Can you work these out from the model? Positions are in its coordinate system, mm. Face numbers are marked on the shaded views. A direction names the side the tool comes from. Give positions to 0.01 mm unless a question says otherwise; leave off trailing zeros. Order: outer loops, then holes, each group sorted by start corner. A loop starts at its lowest first (then second) coordinate and runs counter-clockwise, first axis right, second up. Notation, with made-up numbers: (56, 85.5) - (104, 85.5) arc R28 cw to (104, 110.5) - close; hole circle Ø1 at (31.5, 71.5). An arc over 180 degrees is marked (long way). Write each question's results on one line, items separated by ' | '. Start each with the question number.
from build123d import *

# Parameters (mm, degrees)
BOSS_EXTRUDE1_DEPTH = 25.4
SKETCH2_R           = 6.35
SKETCH2_R_2         = 6.289382054
CUT_EXTRUDE1_DEPTH  = 6.35
SKETCH3_R           = 6.35
CUT_EXTRUDE2_DEPTH  = 65.834626806


with BuildPart() as part:
    # Sketch1 → Boss-Extrude1 (new body)
    with BuildSketch(Plane.XY):
        with BuildLine():
            Line((1.27, 42.381959669), (0, 42.400983542))
            Line((0, 42.400983542), (-1.27, 42.381959669))
            ThreePointArc((-1.27, 42.381959669), (-4.039167101, 38.714670348), (-4.477654975, 34.140282326))
            ThreePointArc((-4.477654975, 34.140282326), (-5.686801313, 32.251452896), (-7.469044916, 33.61281957))
            ThreePointArc((-7.469044916, 33.61281957), (-9.445621582, 37.761366553), (-13.302074292, 40.260380337))
            Line((-13.302074292, 40.260380337), (-14.501990468, 39.843891349))
            Line((-14.501990468, 39.843891349), (-15.688893549, 39.391649173))
            ThreePointArc((-15.688893549, 39.391649173), (-17.036772621, 34.998413532), (-15.884283593, 30.549923177))
            ThreePointArc((-15.884283593, 30.549923177), (-16.374491771, 28.361451696), (-18.514867758, 29.031154701))
            ThreePointArc((-18.514867758, 29.031154701), (-21.7911289, 32.253484654), (-26.269722106, 33.282804957))
            Line((-26.269722106, 33.282804957), (-27.25482686, 32.481037825))
            Line((-27.25482686, 32.481037825), (-28.215474992, 31.650124428))
            ThreePointArc((-28.215474992, 31.650124428), (-27.979491926, 27.060831521), (-25.375033182, 23.274792424))
            ThreePointArc((-25.375033182, 23.274792424), (-25.08717686, 21.050640851), (-27.327524299, 20.947904121))
            ThreePointArc((-27.327524299, 20.947904121), (-31.50830447, 22.855356494), (-36.068853735, 22.290832097))
            Line((-36.068853735, 22.290832097), (-36.720328893, 21.200491771))
            Line((-36.720328893, 21.200491771), (-37.338853735, 20.091127572))
            ThreePointArc((-37.338853735, 20.091127572), (-35.547471572, 15.859313854), (-31.805179274, 13.192378205))
            ThreePointArc((-31.805179274, 13.192378205), (-30.773978173, 11.200812045), (-32.844078098, 10.338027146))
            ThreePointArc((-32.844078098, 10.338027146), (-37.425113508, 10.700535032), (-41.517549284, 8.610255909))
            Line((-41.517549284, 8.610255909), (-41.756817328, 7.362853523))
            Line((-41.756817328, 7.362853523), (-41.958615655, 6.108844216))
            ThreePointArc((-41.958615655, 6.108844216), (-38.827901521, 2.744928878), (-34.399151351, 1.518768476))
            ThreePointArc((-34.399151351, 1.518768476), (-32.748983542, 0), (-34.399151351, -1.518768476))
            ThreePointArc((-34.399151351, -1.518768476), (-38.827901521, -2.744928878), (-41.958615655, -6.108844216))
            Line((-41.958615655, -6.108844216), (-41.756817328, -7.362853523))
            Line((-41.756817328, -7.362853523), (-41.517549284, -8.610255909))
            ThreePointArc((-41.517549284, -8.610255909), (-37.425113508, -10.700535032), (-32.844078098, -10.338027146))
            ThreePointArc((-32.844078098, -10.338027146), (-30.773978173, -11.200812045), (-31.805179274, -13.192378205))
            ThreePointArc((-31.805179274, -13.192378205), (-35.547471572, -15.859313854), (-37.338853735, -20.091127572))
            Line((-37.338853735, -20.091127572), (-36.720328893, -21.200491771))
            Line((-36.720328893, -21.200491771), (-36.068853735, -22.290832097))
            ThreePointArc((-36.068853735, -22.290832097), (-31.50830447, -22.855356494), (-27.327524299, -20.947904121))
            ThreePointArc((-27.327524299, -20.947904121), (-25.08717686, -21.050640851), (-25.375033182, -23.274792424))
            ThreePointArc((-25.375033182, -23.274792424), (-27.979491926, -27.060831521), (-28.215474992, -31.650124428))
            Line((-28.215474992, -31.650124428), (-27.25482686, -32.481037825))
            Line((-27.25482686, -32.481037825), (-26.269722106, -33.282804957))
            ThreePointArc((-26.269722106, -33.282804957), (-21.7911289, -32.253484654), (-18.514867758, -29.031154701))
            ThreePointArc((-18.514867758, -29.031154701), (-16.374491771, -28.361451696), (-15.884283593, -30.549923177))
            ThreePointArc((-15.884283593, -30.549923177), (-17.036772621, -34.998413532), (-15.688893549, -39.391649173))
            Line((-15.688893549, -39.391649173), (-14.501990468, -39.843891349))
            Line((-14.501990468, -39.843891349), (-13.302074292, -40.260380337))
            ThreePointArc((-13.302074292, -40.260380337), (-9.445621582, -37.761366553), (-7.469044916, -33.61281957))
            ThreePointArc((-7.469044916, -33.61281957), (-5.686801313, -32.251452896), (-4.477654975, -34.140282326))
            ThreePointArc((-4.477654975, -34.140282326), (-4.039167101, -38.714670348), (-1.27, -42.381959669))
            Line((-1.27, -42.381959669), (0, -42.400983542))
            Line((0, -42.400983542), (1.27, -42.381959669))
            ThreePointArc((1.27, -42.381959669), (4.039167101, -38.714670348), (4.477654975, -34.140282326))
            ThreePointArc((4.477654975, -34.140282326), (5.686801313, -32.251452896), (7.469044916, -33.61281957))
            ThreePointArc((7.469044916, -33.61281957), (9.445621582, -37.761366553), (13.302074292, -40.260380337))
            Line((13.302074292, -40.260380337), (14.501990468, -39.843891349))
            Line((14.501990468, -39.843891349), (15.688893549, -39.391649173))
            ThreePointArc((15.688893549, -39.391649173), (17.036772621, -34.998413532), (15.884283593, -30.549923177))
            ThreePointArc((15.884283593, -30.549923177), (16.374491771, -28.361451696), (18.514867758, -29.031154701))
            ThreePointArc((18.514867758, -29.031154701), (21.7911289, -32.253484654), (26.269722106, -33.282804957))
            Line((26.269722106, -33.282804957), (27.25482686, -32.481037825))
            Line((27.25482686, -32.481037825), (28.215474992, -31.650124428))
            ThreePointArc((28.215474992, -31.650124428), (27.979491926, -27.060831521), (25.375033182, -23.274792424))
            ThreePointArc((25.375033182, -23.274792424), (25.08717686, -21.050640851), (27.327524299, -20.947904121))
            ThreePointArc((27.327524299, -20.947904121), (31.50830447, -22.855356494), (36.068853735, -22.290832097))
            Line((36.068853735, -22.290832097), (36.720328893, -21.200491771))
            Line((36.720328893, -21.200491771), (37.338853735, -20.091127572))
            ThreePointArc((37.338853735, -20.091127572), (35.547471572, -15.859313854), (31.805179274, -13.192378205))
            ThreePointArc((31.805179274, -13.192378205), (30.773978173, -11.200812045), (32.844078098, -10.338027146))
            ThreePointArc((32.844078098, -10.338027146), (37.425113508, -10.700535032), (41.517549284, -8.610255909))
            Line((41.517549284, -8.610255909), (41.756817328, -7.362853523))
            Line((41.756817328, -7.362853523), (41.958615655, -6.108844216))
            ThreePointArc((41.958615655, -6.108844216), (38.827901521, -2.744928878), (34.399151351, -1.518768476))
            ThreePointArc((34.399151351, -1.518768476), (32.748983542, 0), (34.399151351, 1.518768476))
            ThreePointArc((34.399151351, 1.518768476), (38.827901521, 2.744928878), (41.958615655, 6.108844216))
            Line((41.958615655, 6.108844216), (41.756817328, 7.362853523))
            Line((41.756817328, 7.362853523), (41.517549284, 8.610255909))
            ThreePointArc((41.517549284, 8.610255909), (37.425113508, 10.700535032), (32.844078098, 10.338027146))
            ThreePointArc((32.844078098, 10.338027146), (30.773978173, 11.200812045), (31.805179274, 13.192378205))
            ThreePointArc((31.805179274, 13.192378205), (35.547471572, 15.859313854), (37.338853735, 20.091127572))
            Line((37.338853735, 20.091127572), (36.720328893, 21.200491771))
            Line((36.720328893, 21.200491771), (36.068853735, 22.290832097))
            ThreePointArc((36.068853735, 22.290832097), (31.50830447, 22.855356494), (27.327524299, 20.947904121))
            ThreePointArc((27.327524299, 20.947904121), (25.08717686, 21.050640851), (25.375033182, 23.274792424))
            ThreePointArc((25.375033182, 23.274792424), (27.979491926, 27.060831521), (28.215474992, 31.650124428))
            Line((28.215474992, 31.650124428), (27.25482686, 32.481037825))
            Line((27.25482686, 32.481037825), (26.269722106, 33.282804957))
            ThreePointArc((26.269722106, 33.282804957), (21.7911289, 32.253484654), (18.514867758, 29.031154701))
            ThreePointArc((18.514867758, 29.031154701), (16.374491771, 28.361451696), (15.884283593, 30.549923177))
            ThreePointArc((15.884283593, 30.549923177), (17.036772621, 34.998413532), (15.688893549, 39.391649173))
            Line((15.688893549, 39.391649173), (14.501990468, 39.843891349))
            Line((14.501990468, 39.843891349), (13.302074292, 40.260380337))
            ThreePointArc((13.302074292, 40.260380337), (9.445621582, 37.761366553), (7.469044916, 33.61281957))
            ThreePointArc((7.469044916, 33.61281957), (5.686801313, 32.251452896), (4.477654975, 34.140282326))
            ThreePointArc((4.477654975, 34.140282326), (4.039167101, 38.714670348), (1.27, 42.381959669))
        make_face()
    extrude(amount=BOSS_EXTRUDE1_DEPTH)

    # Sketch2 → Cut-Extrude1 (cut)
    with BuildSketch(Plane.XY.offset(25.4)):
        with Locations((0, 19.05)):
            Circle(SKETCH2_R)
        with Locations((0, -18.989382054)):
            Circle(SKETCH2_R_2)
    cut_extrude1 = extrude(amount=-CUT_EXTRUDE1_DEPTH, mode=Mode.SUBTRACT)

    # Mirror2: Cut-Extrude1 across plane
    add(cut_extrude1.mirror(Plane.XY.offset(12.7)), mode=Mode.SUBTRACT)

    # Sketch3 → Cut-Extrude2 (cut, through all)
    with BuildSketch(Plane(origin=(0, 0, 0), x_dir=(-1, 0, 0), z_dir=(0, 0, -1))):
        Circle(SKETCH3_R)
    extrude(amount=-CUT_EXTRUDE2_DEPTH, mode=Mode.SUBTRACT)


solid = part.part
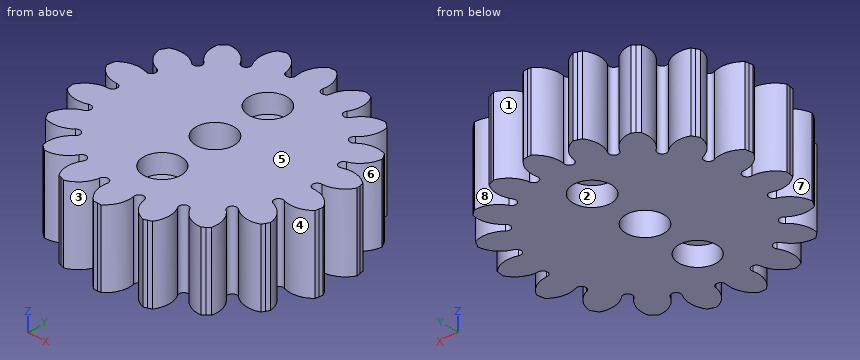
Q1. Which directions (+Z, -Z, +X, -X, +Y, -Y) give clear straight access to the entire face, cutting with the end or side of a thin tool? Please do the marked faces 1, 2, 3 and 4.
Q2. If I drill on probe 1 along X at (y, z) = (37, 4.5); probe 2 along Y at (x, z) = (-1.5, 2.25); probe 3 along Y at (x, z) = (27.5, 15.75), over which ranges is the centre line in solid material (lowest first)? Write a range as from..to.
Q3. If we section it at B-B (y = 19.05): Please give me the cut outline in (x, z), plus the area to 3 significant figures.
Q4. If we section it at C-C (z = 24): State how many separate pieces and enclosed holes the cut face has, plus the area to 3 significant figures.
Q5. Will these pins go through, and if not, where does the flat tip stop? P1, Ø1, axis at x = 30.5, z = 11, coming from the -Y side; P2, Ø6.5, axis at x = 2.5, y = 21, coming from the -Z side; P3, Ø10, axis at y = 20, z = 6, coming from the -X side; P4, Ø2, axis at x = -31, z = 13, coming from the -Y side.
Q6. If we section it at D-D (x = 20.5): Please give me the cut outline in (y, z).
Q7. Thinking about a two-plate mould opening in X: for the marked faces 5, 6, 7 and 8, which applies, released by +X, released by -X, zero draft, split by the parting line, or undercut?
Q8. If we section it at A-A (y = 0): Please give me the cut outline in (x, z).
Findings below:
1) face 1: +Z, -Z, +Y | face 2: -Z | face 3: +Z, -Z, -Y | face 4: +Z, -Z
2) probe 1: x = -16.75..-8.85, -4.51..4.51, 8.85..16.75 | probe 2: y = -42.2..-25.1, -12.88..-6.17, 6.17..12.88, 25.22..42.2 | probe 3: y = -32.27..-25.93, -21.09..21.09, 25.93..32.27
3) outline: (-37.14, 0) - (-6.35, 0) - (-6.35, 6.35) - (6.35, 6.35) - (6.35, 0) - (37.14, 0) - (37.14, 25.4) - (6.35, 25.4) - (6.35, 19.05) - (-6.35, 19.05) - (-6.35, 25.4) - (-37.14, 25.4) - close | area: 1,730 mm2
4) separate pieces: 1 | enclosed holes: 3 | area: 4,360 mm2
5) P1: stops at y = -22.76 | P2: stops at z = 0 | P3: stops at x = -37.34 | P4: stops at y = -22.92
6) outline: (-31.38, 0) - (31.38, 0) - (31.38, 25.4) - (-31.38, 25.4) - close
7) face 5: zero draft | face 6: released by +X | face 7: released by -X | face 8: undercut
8) outline: (-32.75, 0) - (-6.35, 0) - (-6.35, 25.4) - (-32.75, 25.4) - close; (6.35, 0) - (32.75, 0) - (32.75, 25.4) - (6.35, 25.4) - close
